from build123d import *

# Parameters (mm, degrees)
SALIENTE_EXTRUIR1_DEPTH = 15
CROQUIS2_R              = 3.2
CORTAR_EXTRUIR1_DEPTH   = 10.75
CORTAR_EXTRUIR2_START   = -3
CORTAR_EXTRUIR2_DEPTH   = 7.75
CHAFL_N1_SIZE           = 2
SALIENTE_EXTRUIR3_DEPTH = 7.4


with BuildPart() as part:
    # Croquis1 → Saliente-Extruir1 (new body, symmetric)
    with BuildSketch(Plane(origin=(0, 0, 0), x_dir=(1, 0, 0), z_dir=(0, 1, 0))):
        Polygon((0, 0), (-30, 0), (-30, 8), (-1.75, 8), (0, 9.75), (9.4, 9.75), (9.4, 1.75), (0, 1.75), align=None)
    extrude(amount=SALIENTE_EXTRUIR1_DEPTH, both=True)

    # Croquis2 → Cortar-Extruir1 (cut, through all)
    with BuildSketch(Plane.XY):
        with Locations((-15, 0)):
            Circle(CROQUIS2_R)
    extrude(amount=-CORTAR_EXTRUIR1_DEPTH, mode=Mode.SUBTRACT)

    # Croquis3 → Cortar-Extruir2 (cut, through all)
    with BuildSketch(Plane.XY.offset(CORTAR_EXTRUIR2_START)):
        Polygon((-9.226497308, 0), (-12.113248654, 5), (-17.886751346, 5), (-20.773502692, 0), (-17.886751346, -5), (-12.113248654, -5), align=None)
    extrude(amount=-CORTAR_EXTRUIR2_DEPTH, mode=Mode.SUBTRACT)

    # Chaflán1
    chafl_n1_edges = [part.edges().sort_by_distance(p)[0] for p in [
        (9.4, 0, -9.75),
        (9.4, 0, -1.75),
        (-30, 15, -4),
        (-30, -15, -4),
    ]]
    chamfer(chafl_n1_edges, length=CHAFL_N1_SIZE)

    # Croquis5 → Saliente-Extruir3 (add)
    with BuildSketch(Plane(origin=(0, 0, 0), x_dir=(0, 0, -1), z_dir=(1, 0, 0))):
        Polygon((9.75, 12), (10.35, 12), (10.35, 11), (9.75, 10.4), align=None)
        Polygon((9.75, -11), (10.35, -11), (10.35, -12), (9.75, -12.6), align=None)
    extrude(amount=SALIENTE_EXTRUIR3_DEPTH)


solid = part.part
Here's how the part is built. I have some questions about the finished solid (model axes, mm). A direction names the side the tool comes from. Coordinates: 2 decimals unless noted, no trailing zeros. Write each loop counter-clockwise with the first axis right and the second up, starting at its lowest first coordinate (ties: lowest second). Pieces come first, ordered by that corner, then holes. Notation, with made-up numbers: (88, 68) - (125, 68) arc R26 cw to (125, 105) - close; hole circle Ø8 at (34.5, 59). An arc over 180 degrees is marked (long way). Use one line per item in the form item = value.
1) I need wall thicknesses on line 1 (Y direction, x = -15, z = -2.25); line 2 (Y direction, x = -17, z = -3.5); line 3 (Z direction, x = -9, y = -8.5). Which ranges of each line are inside material? Lowest first, please.
Solved:
line_1 = -15 to -3.2, 3.2 to 15
line_2 = -15 to -5, 5 to 15
line_3 = -8 to 0
2) Suppose I cut it at A-A, the plane x = -15. Write out the boundary of the cut face in (y, z), plus the area to 3 significant figures.
Solved:
outline = (-15, -8) - (-5, -8) - (-5, -3) - (-3.2, -3) - (-3.2, 0) - (-15, 0) - close; (3.2, -3) - (5, -3) - (5, -8) - (15, -8) - (15, 0) - (3.2, 0) - close
area = 171 mm2
3) Suppose I cut it at C-C, the plane z = -6.25. Write out the boundary of the cut face in (x, y), plus the area to 3 significant figures.
Solved:
outline = (-30, -13) - (-28, -15) - (9.4, -15) - (9.4, 15) - (-28, 15) - (-30, 13) - close; hole (-20.77, 0) - (-17.89, -5) - (-12.11, -5) - (-9.23, 0) - (-12.11, 5) - (-17.89, 5) - close
area = 1,090 mm2
4) I'm going to push flat-ended pins straight in: P1, Ø1.5, axis at x = 4.5, y = 14, coming from the -Z side; P2, Ø8.5, axis at x = -20, y = 6.5, coming from the -Z side; P3, Ø2.5, axis at x = 3.5, y = -13.5, coming from the -Z side. Where does each tip first touch, or does it pass through?
Solved:
P1 = -9.75
P2 = -8
P3 = -10.1
5) Suppose I cut it at D-D, the plane y = -2. Write out the boundary of the cut face in (x, z).
Solved:
outline = (-30, -8) - (-19.62, -8) - (-19.62, -3) - (-17.5, -3) - (-17.5, 0) - (-30, 0) - close; (-12.5, -3) - (-10.38, -3) - (-10.38, -8) - (-1.75, -8) - (0, -9.75) - (7.4, -9.75) - (9.4, -7.75) - (9.4, -3.75) - (7.4, -1.75) - (0, -1.75) - (0, 0) - (-12.5, 0) - close
6) Thinking about a two-plate mould opening in X: for faces 1 (the flat face through (-15, 5, -5)), 2 (the flat face through (-9, -15, -4)), 3 (the flat face through (-29, -14, -4)), 4 (the flat face through (8.41, -0.21, -2.76)), which applies, released by +X, released by -X, zero draft, split by the parting line, or undercut?
Solved:
face_1 = undercut
face_2 = zero draft
face_3 = released by -X
face_4 = released by +X
7) Suppose I cut it at B-B, the plane y = -11.5. Write out the boundary of the cut face in (x, z), plus the area to 3 significant figures.
Solved:
outline = (-30, -8) - (-1.75, -8) - (0, -9.75) - (0, -10.35) - (7.4, -10.35) - (7.4, -9.75) - (9.4, -7.75) - (9.4, -3.75) - (7.4, -1.75) - (0, -1.75) - (0, 0) - (-30, 0) - close
area = 317 mm2
8) On a 3-axis mill with a long thin cutter (end or side, diameter ignored), from which of +Z, -Z, +X, -X, +Y, -Y can I reach the whole of each face in a straight line? I mean faces 5 (the flat face through (-19, 4, -8)), 6 (the flat face through (4, 14, -9.75)), 7 (the flat face through (4, 0, -9.75)), 8 (the flat face through (-15, -5, -5)). Say none if no direction works.
Solved:
face_5 = -Z, -X, +Y, -Y
face_6 = -Z, +X, -X, +Y
face_7 = -Z, +X, -X
face_8 = -Z
